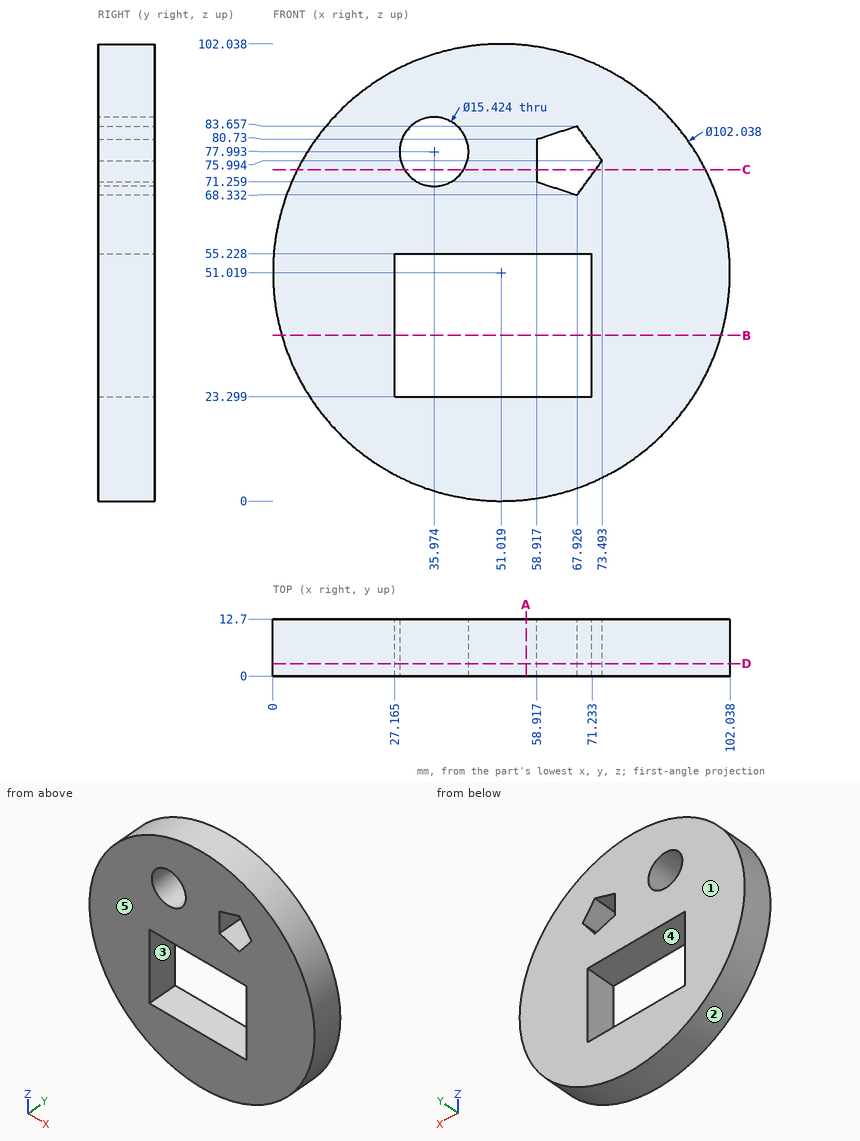
Geometry check sheet. Reference: drawing and pictorial views, mm from the part's lowest x, y, z. A direction names the side the tool comes from. Give positions to 0.01 mm unless a question says otherwise; leave off trailing zeros. Order: outer loops, then holes, each group sorted by start corner. A loop starts at its lowest first (then second) coordinate and runs counter-clockwise, first axis right, second up. Notation, with made-up numbers: M 55,69 L 82,69 A23 ccw 82,81 Z; hole C 86.5,2.25 d4. An arc over 180 degrees is marked long. Answer in a Markdown table with one row per item. Add a question column.
Item 1: Tool access check on the marked faces 4 and 5. Record the directions out of +Z, -Z, +X, -X, +Y, -Y that give a thin tool (end or side, any length) a straight path to the whole face; none if there is none.
Item 2: Section check B-B, the plane z = 37. Enter the section's corners in (x, y) (1 decimal), and give its area (3 significant figures).
Item 3: Gauge pin test, flat ends, axial feed: pin 1 (3 mm diameter, centred on x = 44, y = 8.5, fed in from +Z); pin 2 (1 mm diameter, centred on y = 5.5, z = 92, fed in from +X); pin 3 (6 mm diameter, centred on x = 12.5, y = 6, fed in from +Z). Record the tip position at first contact, or that the pin passes through.
Item 4: Section check D-D, the plane y = 2.75. Enter the section's corners in (x, z) (1 decimal).
Item 5: Mould release check, pull along X, two halves, no side actions. Record for the marked faces 1, 2 and 3: released by +X, released by -X, zero draft, split by the parting line, or undercut.
Item 6: Section check A-A, the plane x = 56.5. Enter the section's corners in (y, z) (1 decimal), and give its area (3 significant figures).
Item 7: Section check C-C, the plane z = 74. Enter the section's corners in (x, y).
Item 8: Scan lines: probe 1 along X at (y, z) = (8.5, 51) (1 decimal); probe 2 along Z at (x, y) = (43, 12.25) (1 decimal); probe 3 along X at (y, z) = (1.5, 77) (1 decimal). Record each from-to range of solid material in increasing order. Write a range as from..to.
Filled sheet:
| question | item | result |
|---|---|---|
| 1 | face 4 | +Y, -Y |
| 1 | face 5 | +Z, -Z, +X, -X, -Y |
| 2 | outline | M 2,0 L 27.2,0 L 27.2,12.7 L 2,12.7 Z; M 71.2,0 L 100.1,0 L 100.1,12.7 L 71.2,12.7 Z |
| 2 | area | 686 mm^2 |
| 3 | pin 1 | stops at z = 101.74 |
| 3 | pin 2 | stops at x = 82.07 |
| 3 | pin 3 | stops at z = 87.64 |
| 4 | outline | C 51,51 d102; hole M 27.2,23.3 L 71.2,23.3 L 71.2,55.2 L 27.2,55.2 Z; hole C 36,78 d15.4; hole M 58.9,71.3 L 67.9,68.3 L 73.5,76 L 67.9,83.7 L 58.9,80.7 Z |
| 5 | face 1 | zero draft |
| 5 | face 2 | split by the parting line |
| 5 | face 3 | undercut |
| 6 | outline | M 0,0.3 L 12.7,0.3 L 12.7,23.3 L 0,23.3 Z; M 0,55.2 L 12.7,55.2 L 12.7,101.7 L 0,101.7 Z |
| 6 | area | 883 mm^2 |
| 7 | outline | M 5.47,0 L 29.38,0 L 29.38,12.7 L 5.47,12.7 Z; M 42.57,0 L 58.92,0 L 58.92,12.7 L 42.57,12.7 Z; M 72.04,0 L 96.57,0 L 96.57,12.7 L 72.04,12.7 Z |
| 8 | probe 1 | x = 0..27.2, 71.2..102 |
| 8 | probe 2 | z = 0.6..23.3, 55.2..74.8, 81.2..101.4 |
| 8 | probe 3 | x = 7.1..28.3, 43.6..58.9, 72.8..94.9 |
